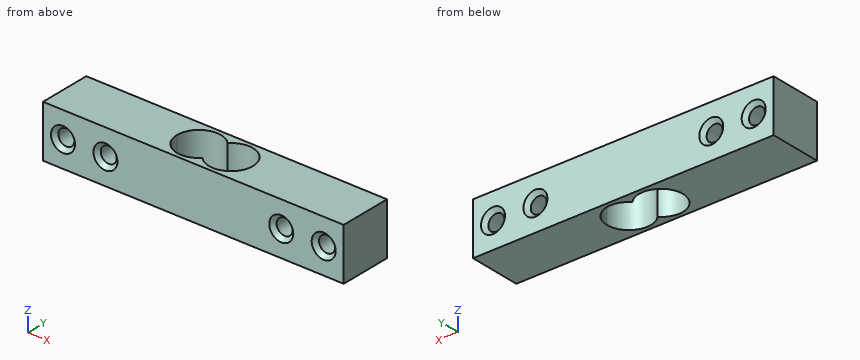
```python
from build123d import *

# Parameters (mm, degrees)
SKETCH1_W           = 75.15
SKETCH1_H           = 13
SKETCH1_R           = 2
BOSS_EXTRUDE1_DEPTH = 13
CHAMFER1_SIZE       = 1
CHAMFER2_SIZE       = 1
CUT_EXTRUDE1_DEPTH  = 13


with BuildPart() as part:
    # Sketch1 → Boss-Extrude1 (new body)
    with BuildSketch(Plane(origin=(0, 0, 0), x_dir=(1, 0, 0), z_dir=(0, 1, 0))):
        with Locations((-2.595641447, 7.241611842)):
            Rectangle(SKETCH1_W, SKETCH1_H)
        with Locations(Location((29.979358553, 7.241611842, 0), (0, 0, 90))):
            Circle(SKETCH1_R, mode=Mode.SUBTRACT)
        with Locations(Location((19.379358553, 7.241611842, 0), (0, 0, 90))):
            Circle(SKETCH1_R, mode=Mode.SUBTRACT)
        with Locations(Location((-35.170641447, 7.241611842, 0), (0, 0, 90))):
            Circle(SKETCH1_R, mode=Mode.SUBTRACT)
        with Locations(Location((-24.570641447, 7.241611842, 0), (0, 0, 90))):
            Circle(SKETCH1_R, mode=Mode.SUBTRACT)
    extrude(amount=BOSS_EXTRUDE1_DEPTH)

    # Chamfer1
    chamfer1_edges = [part.edges().sort_by_distance(p)[0] for p in [
        (19.379358553, 0, -5.241611842),
    ]]
    chamfer(chamfer1_edges, length=CHAMFER1_SIZE)

    # Chamfer2
    chamfer2_edges = [part.edges().sort_by_distance(p)[0] for p in [
        (29.979358553, 0, -5.241611842),
        (29.979358553, 13, -5.241611842),
        (19.379358553, 13, -5.241611842),
        (-35.170641447, 0, -5.241611842),
        (-35.170641447, 13, -5.241611842),
        (-24.570641447, 0, -5.241611842),
        (-24.570641447, 13, -5.241611842),
    ]]
    chamfer(chamfer2_edges, length=CHAMFER2_SIZE)

    # Sketch2 → Cut-Extrude1 (cut)
    with BuildSketch(Plane.XY.offset(-0.741611842)):
        with BuildLine():
            ThreePointArc((-2.595641447, 10.269612049), (-1.48803448, 8.52762176), (-1.100641447, 6.5))
            Line((-1.100641447, 6.5), (6.909358553, 6.5))
            ThreePointArc((6.909358553, 6.5), (3.436980312, 11.612606967), (-2.595641447, 10.269612049))
        make_face()
        with BuildLine():
            ThreePointArc((-2.595641447, 2.730387951), (-1.48803448, 4.47237824), (-1.100641447, 6.5))
            Line((-1.100641447, 6.5), (-4.090641447, 6.5))
            ThreePointArc((-4.090641447, 6.5), (-3.703248414, 4.47237824), (-2.595641447, 2.730387951))
        make_face()
        with BuildLine():
            Line((-4.090641447, 6.5), (-1.100641447, 6.5))
            ThreePointArc((-1.100641447, 6.5), (-1.48803448, 8.52762176), (-2.595641447, 10.269612049))
            ThreePointArc((-2.595641447, 10.269612049), (-3.703248414, 8.52762176), (-4.090641447, 6.5))
        make_face()
        with BuildLine():
            Line((6.909358553, 6.5), (-1.100641447, 6.5))
            ThreePointArc((-1.100641447, 6.5), (-1.48803448, 4.47237824), (-2.595641447, 2.730387951))
            ThreePointArc((-2.595641447, 2.730387951), (3.436980312, 1.387393033), (6.909358553, 6.5))
        make_face()
        with BuildLine():
            ThreePointArc((-2.595641447, 2.730387951), (-3.703248414, 4.47237824), (-4.090641447, 6.5))
            Line((-4.090641447, 6.5), (-12.100641447, 6.5))
            ThreePointArc((-12.100641447, 6.5), (-8.628263207, 1.387393033), (-2.595641447, 2.730387951))
        make_face()
        with BuildLine():
            Line((-12.100641447, 6.5), (-4.090641447, 6.5))
            ThreePointArc((-4.090641447, 6.5), (-3.703248414, 8.52762176), (-2.595641447, 10.269612049))
            ThreePointArc((-2.595641447, 10.269612049), (-8.628263207, 11.612606967), (-12.100641447, 6.5))
        make_face()
    extrude(amount=-CUT_EXTRUDE1_DEPTH, mode=Mode.SUBTRACT)


solid = part.part
```
Part model, mm, in its own coordinate system. Round coordinates to 2 decimals unless told otherwise and drop trailing zeros. Order: outer loops, then holes, each group sorted by start corner. A loop starts at its lowest first (then second) coordinate and runs counter-clockwise, first axis right, second up. Notation, with made-up numbers: M 47,68.5 L 79,68.5 A16 cw 79,78.5 Z; hole C -11,14 d10. An arc over 180 degrees is marked long. Answer in a Markdown table with one row per item. Add a question column.
Q1. Cut at B-B on x = -9. Give the cut face in (y, z).
Q2. Cut at A-A on y = 4. Give the cut face in (x, z), and give its area (3 significant figures).
Q3. Pin check, flat tip, straight feed: pin 1 (2.5 mm diameter, centred on x = -35.17, z = -7.24, fed in from +Y). Stop position of the tip, or through.
Q4. Wall check: L1, parallel to Y at x = -6.5, z = -6.5; L2, parallel to X at y = 4, z = -7; L3, parallel to X at y = 4.5, z = -6.25. Give the ranges that are in metal, low to high. Write a range as from..to.
Q5. Cut at D-D on y = 8.5. Give the cut face in (x, z).
Q6. Cut at C-C on z = -1.75. Give the cut face in (x, y).
Established:
| question | item | result |
|---|---|---|
| 1 | outline | M 0,-13.74 L 1.55,-13.74 L 1.55,-0.74 L 0,-0.74 Z; M 11.45,-13.74 L 13,-13.74 L 13,-0.74 L 11.45,-0.74 Z |
| 2 | outline | M -40.17,-13.74 L -11.5,-13.74 L -11.5,-0.74 L -40.17,-0.74 Z; M 6.31,-13.74 L 34.98,-13.74 L 34.98,-0.74 L 6.31,-0.74 Z; hole C -35.17,-7.24 d4; hole C -24.57,-7.24 d4; hole C 19.38,-7.24 d4; hole C 29.98,-7.24 d4 |
| 2 | area | 695 mm2 |
| 3 | pin 1 | passes through |
| 4 | L1 | y = 0..1, 12..13 |
| 4 | L2 | x = -40.17..-37.16, -33.19..-26.56, -22.59..-11.5, 6.31..17.39, 21.36..27.99, 31.96..34.98 |
| 4 | L3 | x = -40.17..-36.91, -33.43..-26.31, -22.83..-11.72, 6.53..17.64, 21.12..28.24, 31.72..34.98 |
| 5 | outline | M -40.17,-13.74 L -11.72,-13.74 L -11.72,-0.74 L -40.17,-0.74 Z; M 6.53,-13.74 L 34.98,-13.74 L 34.98,-0.74 L 6.53,-0.74 Z; hole C -35.17,-7.24 d4; hole C -24.57,-7.24 d4; hole C 19.38,-7.24 d4; hole C 29.98,-7.24 d4 |
| 6 | outline | M -40.17,0 L 34.98,0 L 34.98,13 L -40.17,13 Z; hole M -2.6,2.73 A5.5 ccw long -2.6,10.27 A5.5 ccw long Z |
